```python
from build123d import *

# Parameters (mm, degrees)
SKETCH1_W           = 38.1
SKETCH1_H           = 91.44
BOSS_EXTRUDE1_DEPTH = 6.35
SKETCH2_W           = 38.1
SKETCH2_H           = 6.35
BOSS_EXTRUDE2_DEPTH = 101.6


with BuildPart() as part:
    # Sketch1 → Boss-Extrude1 (new body)
    with BuildSketch(Plane.XY):
        with Locations((19.05, 45.72)):
            Rectangle(SKETCH1_W, SKETCH1_H)
        with BuildLine():
            Line((33.02, 74.93), (33.02, 11.43))
            ThreePointArc((33.02, 11.43), (30.48, 8.89), (27.94, 11.43))
            Line((27.94, 11.43), (27.94, 74.93))
            ThreePointArc((27.94, 74.93), (30.48, 77.47), (33.02, 74.93))
        make_face(mode=Mode.SUBTRACT)
    extrude(amount=BOSS_EXTRUDE1_DEPTH)

    # Sketch2 → Boss-Extrude2 (add)
    with BuildSketch(Plane.XY.offset(6.35)):
        with Locations((19.05, 3.175)):
            Rectangle(SKETCH2_W, SKETCH2_H)
    extrude(amount=BOSS_EXTRUDE2_DEPTH)


solid = part.part
```
Could you check a few things on this model? Use its own coordinates, in mm. A direction names the side the tool comes from. Round coordinates to 2 decimals unless told otherwise and drop trailing zeros. Order: outer loops, then holes, each group sorted by start corner. A loop starts at its lowest first (then second) coordinate and runs counter-clockwise, first axis right, second up. Notation, with made-up numbers: M -14.5,32.25 L 33.5,32.25 A19 cw 33.5,59.25 Z; hole C 14,-24 d10. An arc over 180 degrees is marked long. One line per question, with ' | ' between items. Start each with the question number.
(1) Suppose I cut it at A-A on x = 30.48. List the corners of the cut face in (y, z) for me.
(2) Suppose I cut it at B-B on y = 59. List the corners of the cut face in (x, z) for me.
(3) Suppose I cut it at C-C on x = 4.5. List the corners of the cut face in (y, z) for me.
(4) Thinking about a two-plate mould opening in Y: for faces 4 (the face through (19, 0, 53)), 5 (the face through (30.54, 8.89, 3.13)), 6 (the face through (19, 91.44, 3)), which applies, +Y half, -Y half, draft (parallel to the pull), parting line (faces both ways), or undercut?
(5) For faces 1 (the face through (19, 6.35, 56)), 2 (the face through (0, 5, 30)), 3 (the face through (27.94, 43, 3)), which set-ups out of +Z, -Z, +X, -X, +Y, -Y let a thin tool reach every point of the face, with its end or its side?
(6) Suppose I cut it at D-D on z = 18. List the corners of the cut face in (x, y) for me.
(7) For P1, Ø8, axis at x = 34, y = 77.5, coming from the -Z side; P2, Ø2, axis at x = 11.5, z = 36, coming from the +Y side; P3, Ø19, axis at x = 23, y = 65.5, coming from the +Z side, each with a flat end and sliding along its axis, tell me the tip position at first contact or that it passes through.
(8) Please list where these lines run through material, in increasing order: line 1 along Y through (x, z) = (29.5, 56.5); line 2 along Y through (x, z) = (31, 6).
Geometry results:
1) outline: M 0,0 L 8.89,0 L 8.89,6.35 L 6.35,6.35 L 6.35,107.95 L 0,107.95 Z; M 77.47,0 L 91.44,0 L 91.44,6.35 L 77.47,6.35 Z
2) outline: M 0,0 L 27.94,0 L 27.94,6.35 L 0,6.35 Z; M 33.02,0 L 38.1,0 L 38.1,6.35 L 33.02,6.35 Z
3) outline: M 0,0 L 91.44,0 L 91.44,6.35 L 6.35,6.35 L 6.35,107.95 L 0,107.95 Z
4) face 4: -Y half | face 5: undercut | face 6: +Y half
5) face 1: +Z, +X, -X, +Y | face 2: +Z, -Z, -X, +Y, -Y | face 3: +Z, -Z
6) outline: M 0,0 L 38.1,0 L 38.1,6.35 L 0,6.35 Z
7) P1: z = 0 | P2: y = 6.35 | P3: z = 6.35
8) line 1: 0 to 6.35 | line 2: 0 to 8.94, 77.42 to 91.44
